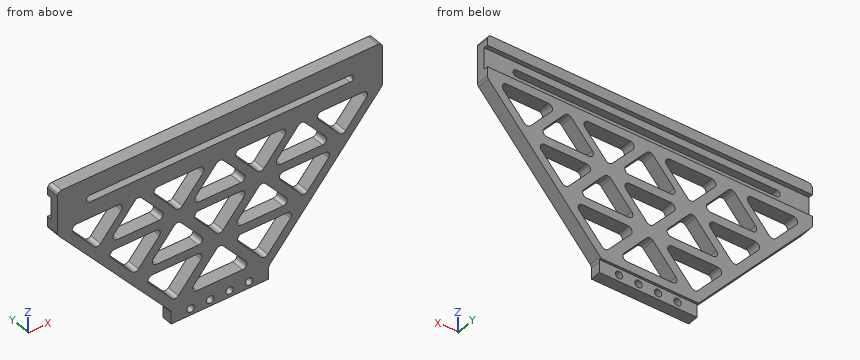
from build123d import *

# Parameters (mm, degrees)
EXTRUDE_1_DEPTH     = 6
SKETCH_2_W          = 150
SKETCH_2_H          = 10
CUT_EXTRUDE_1_DEPTH = 2
SKETCH_3_W          = 45
SKETCH_3_H          = 6
CUT_EXTRUDE_2_DEPTH = 1
HOLE_WIZARD_M31_D   = 3.4
CUT_EXTRUDE_3_DEPTH = 112.937482552
CUT_EXTRUDE_4_REACH = 114.027
FILLET_1_R          = 2


with BuildPart() as part:
    # Эскиз1 → Бобышка-Вытянуть1 (new body)
    with BuildSketch(Plane(origin=(0, 0, 0), x_dir=(1, 0, 0), z_dir=(0, 1, 0))):
        Polygon((-22.5, 3), (22.5, 3), (22.5, -3), (75, -63), (75, -83), (-75, -83), (-75, -63), (-22.5, -3), align=None)
    extrude(amount=EXTRUDE_1_DEPTH)

    # Эскиз2 → Вырез-Вытянуть1 (cut)
    with BuildSketch(Plane(origin=(0, 6, 0), x_dir=(1, 0, 0), z_dir=(0, 1, 0))):
        with Locations((0, -73)):
            Rectangle(SKETCH_2_W, SKETCH_2_H)
    extrude(amount=-CUT_EXTRUDE_1_DEPTH, mode=Mode.SUBTRACT)

    # Эскиз3 → Вырез-Вытянуть2 (cut)
    with BuildSketch(Plane(origin=(0, 6, 0), x_dir=(1, 0, 0), z_dir=(0, 1, 0))):
        Rectangle(SKETCH_3_W, SKETCH_3_H)
    extrude(amount=-CUT_EXTRUDE_2_DEPTH, mode=Mode.SUBTRACT)

    # Отверстие с зазором M31 (through all)
    with Locations(Plane(origin=(0, 0, 0), x_dir=(-1, 0, 0), z_dir=(0, -1, 0))):
        with Locations((-13.5, 0), (-4.5, 0), (4.5, 0), (13.5, 0)):
            Hole(HOLE_WIZARD_M31_D / 2)

    # Эскиз9 → Вырез-Вытянуть3 (cut, through all)
    with BuildSketch(Plane(origin=(0, 4, 0), x_dir=(1, 0, 0), z_dir=(0, 1, 0))):
        with BuildLine():
            Line((-60, -71.4), (60, -71.4))
            ThreePointArc((60, -71.4), (61.6, -73), (60, -74.6))
            Line((60, -74.6), (-60, -74.6))
            ThreePointArc((-60, -74.6), (-61.6, -73), (-60, -71.4))
        make_face()
    extrude(amount=-CUT_EXTRUDE_3_DEPTH, mode=Mode.SUBTRACT)

    # Эскиз10 → Вырез-Вытянуть4 (cut, up to next)
    with BuildSketch(Plane(origin=(0, 6, 0), x_dir=(1, 0, 0), z_dir=(0, 1, 0)), mode=Mode.PRIVATE) as cut_extrude_4_sk1:
        Polygon((-70.559927094, -64), (-56.559927094, -48), (-42.559927094, -64), align=None)
    cut_extrude_4_tool1 = extrude(cut_extrude_4_sk1.sketch, amount=-CUT_EXTRUDE_4_REACH, mode=Mode.PRIVATE) & part.part
    # Эскиз10 → Вырез-Вытянуть4 (cut, up to next)
    with BuildSketch(Plane(origin=(0, 6, 0), x_dir=(1, 0, 0), z_dir=(0, 1, 0)), mode=Mode.PRIVATE) as cut_extrude_4_sk2:
        Polygon((-51.709923067, -48), (-37.709923067, -64), (-23.709923067, -48), align=None)
    cut_extrude_4_tool2 = extrude(cut_extrude_4_sk2.sketch, amount=-CUT_EXTRUDE_4_REACH, mode=Mode.PRIVATE) & part.part
    # Эскиз10 → Вырез-Вытянуть4 (cut, up to next)
    with BuildSketch(Plane(origin=(0, 6, 0), x_dir=(1, 0, 0), z_dir=(0, 1, 0)), mode=Mode.PRIVATE) as cut_extrude_4_sk3:
        Polygon((-18.85991904, -48), (-32.85991904, -64), (-4.85991904, -64), align=None)
    cut_extrude_4_tool3 = extrude(cut_extrude_4_sk3.sketch, amount=-CUT_EXTRUDE_4_REACH, mode=Mode.PRIVATE) & part.part
    # Эскиз10 → Вырез-Вытянуть4 (cut, up to next)
    with BuildSketch(Plane(origin=(0, 6, 0), x_dir=(1, 0, 0), z_dir=(0, 1, 0)), mode=Mode.PRIVATE) as cut_extrude_4_sk4:
        Polygon((-14.009915012, -48), (-0.009915012, -64), (13.990084988, -48), align=None)
    cut_extrude_4_tool4 = extrude(cut_extrude_4_sk4.sketch, amount=-CUT_EXTRUDE_4_REACH, mode=Mode.PRIVATE) & part.part
    # Эскиз10 → Вырез-Вытянуть4 (cut, up to next)
    with BuildSketch(Plane(origin=(0, 6, 0), x_dir=(1, 0, 0), z_dir=(0, 1, 0)), mode=Mode.PRIVATE) as cut_extrude_4_sk5:
        Polygon((18.840089015, -48), (4.840089015, -64), (32.840089015, -64), align=None)
    cut_extrude_4_tool5 = extrude(cut_extrude_4_sk5.sketch, amount=-CUT_EXTRUDE_4_REACH, mode=Mode.PRIVATE) & part.part
    # Эскиз10 → Вырез-Вытянуть4 (cut, up to next)
    with BuildSketch(Plane(origin=(0, 6, 0), x_dir=(1, 0, 0), z_dir=(0, 1, 0)), mode=Mode.PRIVATE) as cut_extrude_4_sk6:
        Polygon((23.690093042, -48), (37.690093042, -64), (51.690093042, -48), align=None)
    cut_extrude_4_tool6 = extrude(cut_extrude_4_sk6.sketch, amount=-CUT_EXTRUDE_4_REACH, mode=Mode.PRIVATE) & part.part
    # Эскиз10 → Вырез-Вытянуть4 (cut, up to next)
    with BuildSketch(Plane(origin=(0, 6, 0), x_dir=(1, 0, 0), z_dir=(0, 1, 0)), mode=Mode.PRIVATE) as cut_extrude_4_sk7:
        Polygon((42.540097069, -64), (70.540097069, -64), (56.540097069, -48), align=None)
    cut_extrude_4_tool7 = extrude(cut_extrude_4_sk7.sketch, amount=-CUT_EXTRUDE_4_REACH, mode=Mode.PRIVATE) & part.part
    # Эскиз10 → Вырез-Вытянуть4 (cut, up to next)
    with BuildSketch(Plane(origin=(0, 6, 0), x_dir=(1, 0, 0), z_dir=(0, 1, 0)), mode=Mode.PRIVATE) as cut_extrude_4_sk8:
        Polygon((-53.059927094, -44), (-39.059927094, -28), (-25.059927094, -44), align=None)
    cut_extrude_4_tool8 = extrude(cut_extrude_4_sk8.sketch, amount=-CUT_EXTRUDE_4_REACH, mode=Mode.PRIVATE) & part.part
    # Эскиз10 → Вырез-Вытянуть4 (cut, up to next)
    with BuildSketch(Plane(origin=(0, 6, 0), x_dir=(1, 0, 0), z_dir=(0, 1, 0)), mode=Mode.PRIVATE) as cut_extrude_4_sk9:
        Polygon((-33.545538953, -28), (-19.545538953, -44), (-5.545538953, -28), align=None)
    cut_extrude_4_tool9 = extrude(cut_extrude_4_sk9.sketch, amount=-CUT_EXTRUDE_4_REACH, mode=Mode.PRIVATE) & part.part
    # Эскиз10 → Вырез-Вытянуть4 (cut, up to next)
    with BuildSketch(Plane(origin=(0, 6, 0), x_dir=(1, 0, 0), z_dir=(0, 1, 0)), mode=Mode.PRIVATE) as cut_extrude_4_sk10:
        Polygon((-0.031150813, -28), (-14.031150813, -44), (13.968849187, -44), align=None)
    cut_extrude_4_tool10 = extrude(cut_extrude_4_sk10.sketch, amount=-CUT_EXTRUDE_4_REACH, mode=Mode.PRIVATE) & part.part
    # Эскиз10 → Вырез-Вытянуть4 (cut, up to next)
    with BuildSketch(Plane(origin=(0, 6, 0), x_dir=(1, 0, 0), z_dir=(0, 1, 0)), mode=Mode.PRIVATE) as cut_extrude_4_sk11:
        Polygon((5.483237327, -28), (19.483237327, -44), (33.483237327, -28), align=None)
    cut_extrude_4_tool11 = extrude(cut_extrude_4_sk11.sketch, amount=-CUT_EXTRUDE_4_REACH, mode=Mode.PRIVATE) & part.part
    # Эскиз10 → Вырез-Вытянуть4 (cut, up to next)
    with BuildSketch(Plane(origin=(0, 6, 0), x_dir=(1, 0, 0), z_dir=(0, 1, 0)), mode=Mode.PRIVATE) as cut_extrude_4_sk12:
        Polygon((24.997625468, -44), (38.997625468, -28), (52.997625468, -44), align=None)
    cut_extrude_4_tool12 = extrude(cut_extrude_4_sk12.sketch, amount=-CUT_EXTRUDE_4_REACH, mode=Mode.PRIVATE) & part.part
    # Эскиз10 → Вырез-Вытянуть4 (cut, up to next)
    with BuildSketch(Plane(origin=(0, 6, 0), x_dir=(1, 0, 0), z_dir=(0, 1, 0)), mode=Mode.PRIVATE) as cut_extrude_4_sk13:
        Polygon((-35.559927094, -24), (-20.684927094, -7), (-5.809927094, -24), align=None)
    cut_extrude_4_tool13 = extrude(cut_extrude_4_sk13.sketch, amount=-CUT_EXTRUDE_4_REACH, mode=Mode.PRIVATE) & part.part
    # Эскиз10 → Вырез-Вытянуть4 (cut, up to next)
    with BuildSketch(Plane(origin=(0, 6, 0), x_dir=(1, 0, 0), z_dir=(0, 1, 0)), mode=Mode.PRIVATE) as cut_extrude_4_sk14:
        Polygon((-14.904785308, -7), (-0.029785308, -24), (14.845214692, -7), align=None)
    cut_extrude_4_tool14 = extrude(cut_extrude_4_sk14.sketch, amount=-CUT_EXTRUDE_4_REACH, mode=Mode.PRIVATE) & part.part
    # Эскиз10 → Вырез-Вытянуть4 (cut, up to next)
    with BuildSketch(Plane(origin=(0, 6, 0), x_dir=(1, 0, 0), z_dir=(0, 1, 0)), mode=Mode.PRIVATE) as cut_extrude_4_sk15:
        Polygon((20.625356478, -7), (5.750356478, -24), (35.500356478, -24), align=None)
    cut_extrude_4_tool15 = extrude(cut_extrude_4_sk15.sketch, amount=-CUT_EXTRUDE_4_REACH, mode=Mode.PRIVATE) & part.part
    add(cut_extrude_4_tool1.solids().sort_by_distance((-56.559927, 6, 58.666667))[0], mode=Mode.SUBTRACT)
    add(cut_extrude_4_tool2.solids().sort_by_distance((-37.709923, 6, 53.333333))[0], mode=Mode.SUBTRACT)
    add(cut_extrude_4_tool3.solids().sort_by_distance((-18.859919, 6, 58.666667))[0], mode=Mode.SUBTRACT)
    add(cut_extrude_4_tool4.solids().sort_by_distance((-0.009915, 6, 53.333333))[0], mode=Mode.SUBTRACT)
    add(cut_extrude_4_tool5.solids().sort_by_distance((18.840089, 6, 58.666667))[0], mode=Mode.SUBTRACT)
    add(cut_extrude_4_tool6.solids().sort_by_distance((37.690093, 6, 53.333333))[0], mode=Mode.SUBTRACT)
    add(cut_extrude_4_tool7.solids().sort_by_distance((56.540097, 6, 58.666667))[0], mode=Mode.SUBTRACT)
    add(cut_extrude_4_tool8.solids().sort_by_distance((-39.059927, 6, 38.666667))[0], mode=Mode.SUBTRACT)
    add(cut_extrude_4_tool9.solids().sort_by_distance((-19.545539, 6, 33.333333))[0], mode=Mode.SUBTRACT)
    add(cut_extrude_4_tool10.solids().sort_by_distance((-0.031151, 6, 38.666667))[0], mode=Mode.SUBTRACT)
    add(cut_extrude_4_tool11.solids().sort_by_distance((19.483237, 6, 33.333333))[0], mode=Mode.SUBTRACT)
    add(cut_extrude_4_tool12.solids().sort_by_distance((38.997625, 6, 38.666667))[0], mode=Mode.SUBTRACT)
    add(cut_extrude_4_tool13.solids().sort_by_distance((-20.684927, 6, 18.333333))[0], mode=Mode.SUBTRACT)
    add(cut_extrude_4_tool14.solids().sort_by_distance((-0.029785, 6, 12.666667))[0], mode=Mode.SUBTRACT)
    add(cut_extrude_4_tool15.solids().sort_by_distance((20.625356, 6, 18.333333))[0], mode=Mode.SUBTRACT)

    # Скругление1
    fillet_1_edges = [part.edges().sort_by_distance(p)[0] for p in [
        (-51.709923067, 3, 48),
        (-23.709923067, 3, 48),
        (-37.709923067, 3, 64),
        (-18.85991904, 3, 48),
        (-4.85991904, 3, 64),
        (-32.85991904, 3, 64),
        (-14.009915012, 3, 48),
        (13.990084988, 3, 48),
        (-0.009915012, 3, 64),
        (75, 3, 63),
        (18.840089015, 3, 48),
        (32.840089015, 3, 64),
        (4.840089015, 3, 64),
        (75, 3, 83),
        (-75, 3, 83),
        (-75, 3, 63),
        (23.690093042, 3, 48),
        (51.690093042, 3, 48),
        (37.690093042, 3, 64),
        (-25.059927094, 3, 44),
        (-53.059927094, 3, 44),
        (-39.059927094, 3, 28),
        (42.540097069, 3, 64),
        (56.540097069, 3, 48),
        (70.540097069, 3, 64),
        (-33.545538953, 3, 28),
        (-5.545538953, 3, 28),
        (-19.545538953, 3, 44),
        (-0.031150813, 3, 28),
        (13.968849187, 3, 44),
        (-14.031150813, 3, 44),
        (5.483237327, 3, 28),
        (33.483237327, 3, 28),
        (19.483237327, 3, 44),
        (52.997625468, 3, 44),
        (24.997625468, 3, 44),
        (38.997625468, 3, 28),
        (-5.809927094, 3, 24),
        (-35.559927094, 3, 24),
        (-20.684927094, 3, 7),
        (-14.904785308, 3, 7),
        (14.845214692, 3, 7),
        (-0.029785308, 3, 24),
        (20.625356478, 3, 7),
        (35.500356478, 3, 24),
        (5.750356478, 3, 24),
        (-22.5, 2.5, 3),
        (22.5, 2.5, 3),
        (-42.559927094, 3, 64),
        (-70.559927094, 3, 64),
        (-56.559927094, 3, 48),
    ]]
    fillet(fillet_1_edges, radius=FILLET_1_R)


solid = part.part
Geometry check sheet. Reference: the model listing, model coordinates, mm. Give positions to 0.01 mm unless a question says otherwise; leave off trailing zeros. Loops run counter-clockwise (first coordinate to the right, second up) from the corner with the lowest first, then second, coordinate; pieces in that order, holes last. Notation, with made-up numbers: (52.25, 35.25) -> (64.25, 35.25) arc R31 cw to (64.25, 68.25) -> close; hole circle Ø11 at (43.25, 67.25). An arc over 180 degrees is marked (long way). Answer in a Markdown table with one row per item. Add a question column.
1) Cross-section at A-A on z = 73. Record the boundary of the cut face in (x, y).
2) Gauge pin test, flat ends, axial feed: P1, Ø1.1, axis at x = -5.5, y = 5.5, coming from the -Z side; P2, Ø2, axis at x = -4.5, z = 0, coming from the -Y side; P3, Ø1.8, axis at x = 38, y = 2, coming from the -Z side; P4, Ø2.5, axis at y = 3.5, z = -0.5, coming from the +X side. Record the tip position at first contact, or that the pin passes through.
3) Cross-section at B-B on z = 0. Record the boundary of the cut face in (x, y), and give its area (3 significant figures).
4) Material ranges on probe 1 along Z at (x, y) = (38, 2); probe 2 along Z at (x, y) = (-4.5, 1.25); probe 3 along Z at (x, y) = (-13.5, 3), recorded low to high. Write a range as from..to.
5) Cross-section at C-C on x = 4.5. State how many separate pieces and enclosed holes the cut face has, and give its area (3 significant figures).
Outcome:
| question | item | result |
|---|---|---|
| 1 | outline | (-75, 0) -> (-61.6, 0) -> (-61.6, 4) -> (-75, 4) -> close; (61.6, 0) -> (75, 0) -> (75, 4) -> (61.6, 4) -> close |
| 2 | P1 | stops at z = -3 |
| 2 | P2 | passes through |
| 2 | P3 | stops at z = 19.69 |
| 2 | P4 | stops at x = 22.5 |
| 3 | outline | (-22.5, 0) -> (-15.2, 0) -> (-15.2, 5) -> (-22.5, 5) -> close; (-11.8, 0) -> (-6.2, 0) -> (-6.2, 5) -> (-11.8, 5) -> close; (-2.8, 0) -> (2.8, 0) -> (2.8, 5) -> (-2.8, 5) -> close; (6.2, 0) -> (11.8, 0) -> (11.8, 5) -> (6.2, 5) -> close; (15.2, 0) -> (22.5, 0) -> (22.5, 5) -> (15.2, 5) -> close |
| 3 | area | 157 mm^2 |
| 4 | probe 1 | z = 20.71..29.3, 44..48, 62.94..71.4, 74.6..83 |
| 4 | probe 2 | z = -3..-1.7, 1.7..7, 18.89..33.11, 44..48, 58.87..71.4, 74.6..83 |
| 4 | probe 3 | z = -3..-1.7, 1.7..15.21, 24..28, 37.09..54.13, 64..71.4, 74.6..83 |
| 5 | separate pieces | 6 |
| 5 | enclosed holes | 0 |
| 5 | area | 259 mm^2 |
